Autodesk Inventor part; units mm, degrees
ref_plane "YZ Plane" through (0, 0, 0) normal (1, 0, 0) x (0, 1, 0)
ref_plane "XZ Plane" through (0, 0, 0) normal (0, 1, 0) x (-1, 0, 0)
ref_plane "XY Plane" through (0, 0, 0) normal (0, 0, 1) x (1, 0, 0)
sketch "Sketch3" plane through (0, 0, 0) normal (0, 0, 1) x (1, 0, 0)
  line L0 (12.7, -12.7) -> (-12.7, -12.7)
  line L1 (-12.7, -12.7) -> (-12.7, 12.7)
  line L2 (-12.7, 12.7) -> (12.7, 12.7)
  line L3 (12.7, 12.7) -> (12.7, -12.7)
  line L4 (12.7, -12.7) -> (-12.7, 12.7) construction
  line L5 (-12.7, -12.7) -> (12.7, 12.7) construction
  point P0 (0, 0)
  dimension "d0" = 25.4
  dimension "d1" = 25.4
extrude "Cubo" add sketch "Sketch3" along normal blind 25.4
sketch "Sketch5" plane through (0, 0, 25.4) normal (0, 0, 1) x (1, 0, 0)
  line L0 (-12.1868, 12.0555) -> (12.0292, 12.0555) construction
  line L1 (12.0292, 12.0555) -> (12.0292, -12.3181) construction
  line L2 (12.0292, -12.3181) -> (-12.1868, -12.3181) construction
  line L3 (-12.1868, -12.3181) -> (-12.1868, 12.0555) construction
  line L4 (9.4966, -10.2913) -> (5.7916, -10.2913)
  line L5 (5.7916, -10.2913) -> (-0.1365, -2.1567)
  line L6 (-0.1365, -2.1567) -> (-6.1633, -10.2913)
  line L7 (-6.1633, -10.2913) -> (-9.6707, -10.2913)
  line L8 (-9.6707, -10.2913) -> (-1.9149, -0.1313)
  line L9 (-1.9149, -0.1313) -> (-9.4402, 10.0287)
  line L10 (-9.4402, 10.0287) -> (-5.7352, 10.0287)
  line L11 (-5.7352, 10.0287) -> (0.0776, 2.0588)
  line L12 (0.0776, 2.0588) -> (5.9892, 10.0287)
  line L13 (5.9892, 10.0287) -> (9.4966, 10.0287)
  line L14 (9.4966, 10.0287) -> (1.856, 0.0169)
  line L15 (1.856, 0.0169) -> (9.4966, -10.2913)
  point P0 (0, 0)
extrude "X" cut sketch "Sketch5" against normal blind 3.175
sketch "Sketch6" plane through (12.7, -12.7, 0) normal (1, 0, 0) x (0, 0, -1)
  line L0 (-25.0445, 24.9615) -> (-0.3507, 24.9615) construction
  line L1 (-0.3507, 24.9615) -> (-0.3507, 0.3203) construction
  line L2 (-0.3507, 0.3203) -> (-25.0445, 0.3203) construction
  line L3 (-25.0445, 0.3203) -> (-25.0445, 24.9615) construction
  line L4 (-4.069, 2.4809) -> (-21.0792, 2.4809)
  line L5 (-21.0792, 2.4809) -> (-21.0792, 5.0003)
  line L6 (-21.0792, 5.0003) -> (-8.0375, 20.3967)
  line L7 (-8.0375, 20.3967) -> (-20.4864, 20.3967)
  line L8 (-20.4864, 20.3967) -> (-20.4864, 22.8009)
  line L9 (-20.4864, 22.8009) -> (-4.3984, 22.8009)
  line L10 (-4.3984, 22.8009) -> (-4.3984, 20.3638)
  line L11 (-4.3984, 20.3638) -> (-17.5718, 4.885)
  line L12 (-17.5718, 4.885) -> (-4.069, 4.885)
  line L13 (-4.069, 4.885) -> (-4.069, 2.4809)
  point P0 (0, 12.7)
extrude "Z" cut sketch "Sketch6" against normal blind 3.175
sketch "Sketch7" plane through (0, 0, 0) normal (0, 0, -1) x (-1, 0, 0)
  line L0 (-12.3672, 12.2796) -> (12.4407, 12.2796) construction
  line L1 (12.4407, 12.2796) -> (12.4407, -12.4691) construction
  line L2 (12.4407, -12.4691) -> (-12.3672, -12.4691) construction
  line L3 (-12.3672, -12.4691) -> (-12.3672, 12.2796) construction
  line L4 (-1.8683, -10.2547) -> (-1.8683, -1.7055)
  line L5 (-1.8683, -1.7055) -> (-8.559, 10.0653)
  line L6 (-8.559, 10.0653) -> (-4.2379, 10.0653)
  line L7 (-4.2379, 10.0653) -> (0.0677, 2.0116)
  line L8 (0.0677, 2.0116) -> (4.2959, 10.0653)
  line L9 (4.2959, 10.0653) -> (8.555, 10.0653)
  line L10 (8.555, 10.0653) -> (1.8178, -1.7364)
  line L11 (1.8178, -1.7364) -> (1.8178, -10.2547)
  line L12 (1.8178, -10.2547) -> (-1.8683, -10.2547)
  point P0 (0, 0)
extrude "Y" cut sketch "Sketch7" against normal blind 3.175
properties part number "Cubo_3DPrint"
Verification items for the finished model (mm, model axes). A direction names the side the tool comes from. Give positions to 0.01 mm unless a question says otherwise; leave off trailing zeros. Write each loop counter-clockwise with the first axis right and the second up, starting at its lowest first coordinate (ties: lowest second). Pieces come first, ordered by that corner, then holes. Notation, with made-up numbers: (58.25, 82) - (103.25, 82) arc R28 cw to (103.25, 116) - close; hole circle Ø1 at (80.25, 16). An arc over 180 degrees is marked (long way). Answer as CSV lines item,"result". Start each with the question number.
1. Set-up check for faces 4 (the face through (5.17, 4.1, 1.57)), 5 (the face through (11.135, 0.033, 10.893)), 6 (the face through (0, 12.7, 13)), 7 (the face through (5.73, 5.09, 23.83)): record each of +Z, -Z, +X, -X, +Y, -Y from which the full face is reachable in a straight line by a thin tool's end or side.
2. Thickness scan on line 1 (Y direction, x = 11, z = 7.75) (3 decimals); line 2 (X direction, y = 4, z = 2.75); line 3 (Y direction, x = 10.25, z = 6.5) (3 decimals). Record the ranges inside material, lowest first.
3. Draft check along X on faces 1 (the face through (11, 9, 4.398)), 2 (the face through (3, 6, 24)), 3 (the face through (12.7, 0, 10)). Enter one of: pulls with the +X half, pulls with the -X half, needs draft (parallel to the pull), parting line crosses it, or undercut.
4. Sectioned sample at A-A (y = -0.5). Record the boundary of the cut face in (x, z) (3 decimals).
5. Sectioned sample at C-C (x = -1.25). Record the boundary of the cut face in (y, z) (3 decimals), then the cut area to 3 significant figures.
6. Sectioned sample at D-D (y = -4.5). Record the boundary of the cut face in (x, z) (3 decimals), then the cut area to 3 significant figures.
7. Sectioned sample at B-B (z = 13.75). Record the boundary of the cut face in (x, y) (3 decimals).
Derived:
1,face 4,"-Z"
1,face 5,"+X"
1,face 6,"+Z, -Z, +X, -X, +Y"
1,face 7,"+Z"
2,line 1,"-12.7 to -10.219, -7.815 to 3.726, 10.101 to 12.7"
2,line 2,"-12.7 to -5.09, -1.11 to 1, 5.11 to 12.7"
2,line 3,"-12.7 to -10.219, -7.815 to 5.194, 10.101 to 12.7"
3,face 1,"needs draft"
3,face 2,"undercut"
3,face 3,"pulls with the +X half"
4,outline,"(-12.7, 0) - (-2.524, 0) - (-2.524, 3.175) - (2.554, 3.175) - (2.554, 0) - (12.7, 0) - (12.7, 11.346) - (9.525, 11.346) - (9.525, 14.981) - (12.7, 14.981) - (12.7, 25.4) - (2.239, 25.4) - (2.239, 22.225) - (-2.196, 22.225) - (-2.196, 25.4) - (-12.7, 25.4) - close"
5,outline,"(-12.7, 0) - (-10.255, 0) - (-10.255, 3.175) - (4.264, 3.175) - (4.264, 0) - (12.7, 0) - (12.7, 25.4) - (3.879, 25.4) - (3.879, 22.225) - (-3.66, 22.225) - (-3.66, 25.4) - (-12.7, 25.4) - close"
5,area,"575 mm²"
6,outline,"(-12.7, 0) - (-1.818, 0) - (-1.818, 3.175) - (1.868, 3.175) - (1.868, 0) - (12.7, 0) - (12.7, 14.751) - (9.525, 14.751) - (9.525, 18.369) - (12.7, 18.369) - (12.7, 25.4) - (5.204, 25.4) - (5.204, 22.225) - (1.571, 22.225) - (1.571, 25.4) - (-1.873, 25.4) - (-1.873, 22.225) - (-5.25, 22.225) - (-5.25, 25.4) - (-12.7, 25.4) - close"
6,area,"600 mm²"
7,outline,"(-12.7, -12.7) - (12.7, -12.7) - (12.7, -10.219) - (9.525, -10.219) - (9.525, -7.815) - (12.7, -7.815) - (12.7, -3.324) - (9.525, -3.324) - (9.525, 0.953) - (12.7, 0.953) - (12.7, 7.697) - (9.525, 7.697) - (9.525, 10.101) - (12.7, 10.101) - (12.7, 12.7) - (-12.7, 12.7) - close"
